Here's how the part is built. I have some questions about the finished solid (model axes, mm). Face numbers are marked on the shaded views. A direction names the side the tool comes from. Round coordinates to 2 decimals unless told otherwise and drop trailing zeros. Order: outer loops, then holes, each group sorted by start corner. A loop starts at its lowest first (then second) coordinate and runs counter-clockwise, first axis right, second up. Notation, with made-up numbers: M -3,87 L 44,87 A31 ccw 44,121 Z; hole C -15.75,-7 d10. An arc over 180 degrees is marked long. Write item = value, one per line. Start each with the question number.
Item 1: For the marked faces 1, 2 and 3, which set-ups out of +Z, -Z, +X, -X, +Y, -Y let a thin tool reach every point of the face, with its end or its side?
Item 2: I want a section at C-C, the plane y = -66.5. List the corners of the cut face in (x, z) for me.
Item 3: I want a section at B-B, the plane z = 52.5. List the corners of the cut face in (x, y) for me, plus the area to 3 significant figures.
Item 4: We'd pull the mould along X, two halves only. Please class the marked faces 4, 5 and 6: pulls with the +X half, pulls with the -X half, needs draft (parallel to the pull), parting line crosses it, or undercut.
Item 5: I want a section at D-D, the plane x = 23.5. List the corners of the cut face in (y, z) for me.
Item 6: I'm going to push flat-ended pins straight in: P1, Ø4, axis at y = 17.5, z = 19.5, coming from the -X side; P2, Ø3.5, axis at x = 23.5, z = 5.5, coming from the +Y side; P3, Ø17.5, axis at y = 11.5, z = 21.5, coming from the +X side; P4, Ø6.5, axis at x = -23.5, z = 52.5, coming from the +Y side. Where does each tip first touch, or does it pass through?
Item 7: Please list where these lines run through material, in increasing order: L1, parallel to Y at x = 69, z = 29; L2, parallel to X at y = 51.35, z = 52.5; L3, parallel to X at y = 15, z = 15.
Item 8: I want a section at A-A, the plane x = 0. List the corners of the cut face in (y, z) for me.
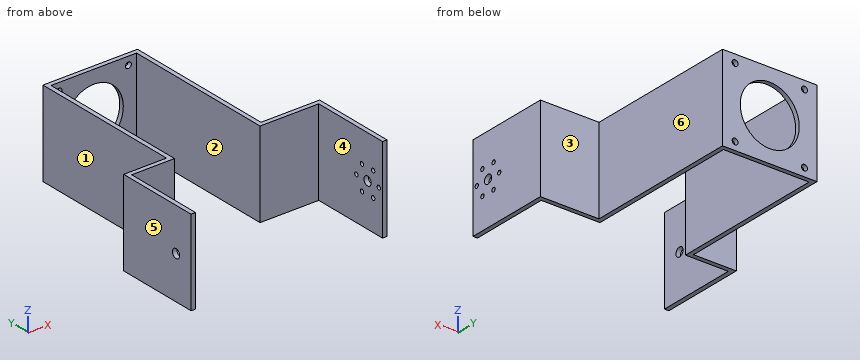
```python
from build123d import *

# Parameters (mm, degrees)
BOSS_EXTRUDE1_DEPTH = 58
SKETCH3_R           = 2
SKETCH3_R_2         = 20
CUT_EXTRUDE1_DEPTH  = 58
SKETCH4_R           = 3
SKETCH4_R_2         = 1.4
CUT_EXTRUDE2_DEPTH  = 58
SKETCH5_R           = 3
CUT_EXTRUDE3_DEPTH  = 58


with BuildPart() as part:
    # Sketch2 → Boss-Extrude1 (new body)
    with BuildSketch(Plane.XY):
        Polygon((0, 51.896715462), (32, 51.896715462), (32, -52.603284538), (71.75, -52.603284538), (71.75, -109.603284538), (68.75, -109.603284538), (68.75, -55.603284538), (29, -55.603284538), (29, 48.896715462), (0, 48.896715462), (-29, 48.896715462), (-29, -55.603284538), (-58, -55.603284538), (-58, -109.603284538), (-61, -109.603284538), (-61, -52.603284538), (-32, -52.603284538), (-32, 51.896715462), align=None)
    extrude(amount=BOSS_EXTRUDE1_DEPTH)

    # Sketch3 → Cut-Extrude1 (cut)
    with BuildSketch(Plane(origin=(0, 51.896715462, 0), x_dir=(1, 0, 0), z_dir=(0, 1, 0))):
        with Locations((-23.5, -5.5)):
            Circle(SKETCH3_R)
        with Locations((23.5, -5.5)):
            Circle(SKETCH3_R)
        with Locations((23.5, -52.5)):
            Circle(SKETCH3_R)
        with Locations((-23.5, -52.5)):
            Circle(SKETCH3_R)
        with Locations((0, -29)):
            Circle(SKETCH3_R_2)
    extrude(amount=-CUT_EXTRUDE1_DEPTH, mode=Mode.SUBTRACT)

    # Sketch4 → Cut-Extrude2 (cut)
    with BuildSketch(Plane(origin=(71.75, 0, 0), x_dir=(0, 0, -1), z_dir=(1, 0, 0))):
        with Locations((-29, -96.903284538)):
            Circle(SKETCH4_R)
        with Locations((-29, -87.403284538)):
            Circle(SKETCH4_R_2)
        with Locations((-20.772758664, -92.153284538)):
            Circle(SKETCH4_R_2)
        with Locations((-20.772758664, -101.653284538)):
            Circle(SKETCH4_R_2)
        with Locations((-29, -106.403284538)):
            Circle(SKETCH4_R_2)
        with Locations((-37.227241336, -101.653284538)):
            Circle(SKETCH4_R_2)
        with Locations((-37.227241336, -92.153284538)):
            Circle(SKETCH4_R_2)
    extrude(amount=-CUT_EXTRUDE2_DEPTH, mode=Mode.SUBTRACT)

    # Sketch5 → Cut-Extrude3 (cut)
    with BuildSketch(Plane.ZY.offset(61)):
        with Locations((29, -96.903284538)):
            Circle(SKETCH5_R)
    extrude(amount=-CUT_EXTRUDE3_DEPTH, mode=Mode.SUBTRACT)


solid = part.part
```
Filled in:
q1.face_1 = +Z, -Z, -X, +Y
q1.face_2 = +Z, -Z, -Y
q1.face_3 = +Z, -Z, +X, +Y
q2.outline = M -61,0 L -58,0 L -58,58 L -61,58 Z; M 68.75,0 L 71.75,0 L 71.75,58 L 68.75,58 Z
q3.outline = M -61,-109.6 L -58,-109.6 L -58,-55.6 L -29,-55.6 L -29,48.9 L -25.5,48.9 L -25.5,51.9 L -32,51.9 L -32,-52.6 L -61,-52.6 Z; M -21.5,48.9 L 21.5,48.9 L 21.5,51.9 L -21.5,51.9 Z; M 25.5,48.9 L 29,48.9 L 29,-55.6 L 68.75,-55.6 L 68.75,-109.6 L 71.75,-109.6 L 71.75,-52.6 L 32,-52.6 L 32,51.9 L 25.5,51.9 Z
q3.area = 1,330 mm^2
q4.face_4 = undercut
q4.face_5 = pulls with the -X half
q4.face_6 = pulls with the +X half
q5.outline = M 48.9,0 L 51.9,0 L 51.9,3.5 L 48.9,3.5 Z; M 48.9,7.5 L 51.9,7.5 L 51.9,50.5 L 48.9,50.5 Z; M 48.9,54.5 L 51.9,54.5 L 51.9,58 L 48.9,58 Z
q6.P1 = -32
q6.P2 = through
q6.P3 = 32
q6.P4 = 51.9
q7.L1 = -109.6 to -107.8, -105 to -99.9, -93.9 to -88.8, -86 to -52.6
q7.L2 = -32 to -25.5, -21.5 to 21.5, 25.5 to 32
q7.L3 = -32 to -29, 29 to 32
q8.outline = M 48.9,0 L 51.9,0 L 51.9,9 L 48.9,9 Z; M 48.9,49 L 51.9,49 L 51.9,58 L 48.9,58 Z
